The model under review builds one solid part; all positions refer to its coordinate system, in mm. A direction names the side the tool comes from. Round coordinates to 2 decimals unless told otherwise and drop trailing zeros. Loops run counter-clockwise (first coordinate to the right, second up) from the corner with the lowest first, then second, coordinate; pieces in that order, holes last. Notation, with made-up numbers: M 1,7.5 L 58,7.5 A16 ccw 58,28.5 Z; hole C 56,78.5 d6. An arc over 180 degrees is marked long. Return JSON: item names as keys, results as strings. Group by question number.
Q1. Consider section C-C (z = 11). State the section outline as (x, y) points.
Q2. For faces 1 (the face through (9, -1, 5)), 2 (the face through (65, -93, 29.818)), 3 (the face through (9, -1, 0)), list the 3-axis set-ups (+Z, -Z, +X, -X, +Y, -Y) from which the entire face can be reached by the end or side of a thin tool; tool diameter is ignored.
Q3. To check wall thickness, follow line 1 along Z through (x, y) = (-3, -10); line 2 along X through (y, z) = (30, 19); line 3 along X through (y, z) = (62, 19). State the ranges of each line that lie inside material, in increasing order.
Q4. Clearance check with flat-ended pins moving along their axes: pin 1 Ø12 at (y, z) = (70.5, 13) entering from -X; pin 2 Ø2 at (y, z) = (13.5, 9.5) entering from +X; pin 3 Ø12 at (y, z) = (12, 24.5) entering from +X. State where each tip first meets the part, or that it passes through.
Q5. Consider section B-B (x = 10). State the section outline as (y, z) points, and give its area (3 significant figures).
Q6. Consider section A-A (y = 0). State the section outline as (x, z) points, and give its area (3 significant figures).
Autodesk Inventor part; units mm, degrees
ref_plane "YZ Plane" through (0, 0, 0) normal (1, 0, 0) x (0, 1, 0)
ref_plane "XZ Plane" through (0, 0, 0) normal (0, 1, 0) x (-1, 0, 0)
ref_plane "XY Plane" through (0, 0, 0) normal (0, 0, 1) x (1, 0, 0)
sketch "Boceto3" plane through (0, 0, 0) normal (0, 0, 1) x (1, 0, 0)
  line L0 (0, 0) -> (82.3331, 0)
  line L1 (86.4856, 2.2148) -> (103.5144, 27.6027)
  line L2 (107.6669, 29.8175) -> (125, 29.8175)
  line L3 (125, 29.8175) -> (125, 34.8175)
  line L4 (125, 34.8175) -> (102.6669, 34.8175)
  line L5 (98.5144, 32.6027) -> (81.4856, 7.2148)
  line L6 (77.3331, 5) -> (0, 5)
  line L7 (0, 5) -> (0, 0)
  arc A0 (77.3331, 5) -> (81.4856, 7.2148) centre (77.3331, 10) ccw
  arc A1 (102.6669, 34.8175) -> (98.5144, 32.6027) centre (102.6669, 29.8175) ccw
  arc A2 (107.6669, 29.8175) -> (103.5144, 27.6027) centre (107.6669, 24.8175) ccw
  arc A3 (82.3331, 0) -> (86.4856, 2.2148) centre (82.3331, 5) ccw
  point P0 (85, 0)
  point P1 (100, 34.8175)
  point P2 (80, 5)
  dimension "d6" = 125
  dimension "d8" = 80
  dimension "d9" = 5
  dimension "d10" = 5
  dimension "d12" = 100
  dimension "d13" = 85
  dimension "d16" = 5
  dimension "d17" = 5
revolve "Revolución1" add sketch "Boceto3" angle 360 about axis through (0, 5, 0) along (0, -1, 0)
move or copy body "Desplazar cuerpo1" bodies to move or copy 1 copy no rotation origin (0, 0, 0) rotation axis (1, 0, 0) rotation angle 90
move or copy body "Desplazar cuerpo2" bodies to move or copy 1 copy no translate (10, 0, 0)
properties part number "plato" material "Porcelana, marfil"
Values:
{
 "1": {"outline": "C 10,0 d184.76; hole C 10,0 d168.05"},
 "2": {"face 1": "+Z", "face 2": "-Z", "face 3": "-Z, +X, -X, +Y, -Y"},
 "3": {"line 1": "z = 0 to 5", "line 2": "x = -83.03 to -74.21, 94.21 to 103.03", "line 3": "x = -65.56 to -54.39, 74.39 to 85.56"},
 "4": {"pin 1": "stops at x = -60.25", "pin 2": "stops at x = 101.06", "pin 3": "stops at x = 134.66"},
 "5": {"outline": "M -125,29.82 L -107.67,29.82 A5 cw -103.51,27.6 L -86.49,2.21 A5 ccw -82.33,0 L 82.33,0 A5 ccw 86.49,2.21 L 103.51,27.6 A5 cw 107.67,29.82 L 125,29.82 L 125,34.82 L 102.67,34.82 A5 ccw 98.51,32.6 L 81.49,7.21 A5 cw 77.33,5 L -77.33,5 A5 cw -81.49,7.21 L -98.51,32.6 A5 ccw -102.67,34.82 L -125,34.82 Z", "area": "1,550 mm2"},
 "6": {"outline": "M -115,29.82 L -97.67,29.82 A5 cw -93.51,27.6 L -76.49,2.21 A5 ccw -72.33,0 L 92.33,0 A5 ccw 96.49,2.21 L 113.51,27.6 A5 cw 117.67,29.82 L 135,29.82 L 135,34.82 L 112.67,34.82 A5 ccw 108.51,32.6 L 91.49,7.21 A5 cw 87.33,5 L -67.33,5 A5 cw -71.49,7.21 L -88.51,32.6 A5 ccw -92.67,34.82 L -115,34.82 Z", "area": "1,550 mm2"}
}
